from build123d import *

# Parameters (mm, degrees)
SKETCH1_W               = 50
SKETCH1_H               = 6
BOSS_EXTRUDE1_DEPTH     = 8
SKETCH2_W               = 15
SKETCH2_H               = 6
CUT_EXTRUDE1_DEPTH      = 3.1
CUT_EXTRUDE2_DEPTH      = 27.419689627
CUT_EXTRUDE2_DEPTH_BACK = 27.419689627
SKETCH3_R               = 1.6
FILLET1_R               = 2.5


with BuildPart() as part:
    # Sketch1 → Boss-Extrude1 (new, symmetric)
    with BuildSketch(Plane(origin=(0, 0, 0), x_dir=(1, 0, 0), z_dir=(0, 1, 0))):
        Rectangle(SKETCH1_W, SKETCH1_H)
    extrude(amount=BOSS_EXTRUDE1_DEPTH, both=True)

    # Sketch2 → Cut-Extrude1 (cut, symmetric)
    with BuildSketch(Plane(origin=(0, 0, 0), x_dir=(1, 0, 0), z_dir=(0, 1, 0))):
        Polygon((-25, -3), (-10, -3), (-17.736081979, 3), (-25, 3), align=None)
        with Locations((17.5, 0)):
            Rectangle(SKETCH2_W, SKETCH2_H)
        Polygon((5, 3), (-14.736081979, 3), (-7, -3), (5, -3), align=None)
    extrude(amount=CUT_EXTRUDE1_DEPTH, both=True, mode=Mode.SUBTRACT)

    # Sketch3 → Cut-Extrude2 (cut, two sides: drawn at the far end of the back side and taken through both)
    with BuildSketch(Plane(origin=(0, 0, 0), x_dir=(1, 0, 0), z_dir=(0, 1, 0)).offset(-CUT_EXTRUDE2_DEPTH_BACK)):
        with Locations(Location((-22, 0, 0), (0, 0, 270))):
            Circle(SKETCH3_R)
        with Locations(Location((22, 0, 0), (0, 0, 270))):
            Circle(SKETCH3_R)
        with Locations(Location((-2.5, 0, 0), (0, 0, 270))):
            Circle(SKETCH3_R)
    extrude(amount=CUT_EXTRUDE2_DEPTH + CUT_EXTRUDE2_DEPTH_BACK, mode=Mode.SUBTRACT)

    # Fillet1
    fillet1_edges = [part.edges().sort_by_distance(p)[0] for p in [
        (25, -5.55, 3),
        (-25, -5.55, 3),
        (-25, -5.55, -3),
        (25, -5.55, -3),
        (5, 0, -3),
        (5, 0, 3),
        (-14.736081979, 0, -3),
        (10, 0, 3),
        (10, 0, -3),
        (-10, 0, 3),
        (25, 5.55, 3),
        (-25, 5.55, 3),
        (-25, 5.55, -3),
        (25, 5.55, -3),
    ]]
    fillet(fillet1_edges, radius=FILLET1_R - 0.0001)  # a hair under: the kernel refuses the full size


solid = part.part
Work out the finished part from the listing and answer in its coordinate system (mm). A direction names the side the tool comes from. Coordinates: 2 decimals unless noted, no trailing zeros. Write each loop counter-clockwise with the first axis right and the second up, starting at its lowest first coordinate (ties: lowest second). Pieces come first, ordered by that corner, then holes. Notation, with made-up numbers: (2.25, 86.25) - (27.25, 86.25) arc R25 cw to (27.25, 112.25) - close; hole circle Ø8 at (-20, 43). An arc over 180 degrees is marked (long way). One line per question, with ' | ' between items.
1) Consider probe 1 along X at (y, z) = (6.4, 0); probe 2 along Z at (x, y) = (22, 6.4); probe 3 along Y at (x, z) = (-12.5, 2.25). Determine where each line is inside the solid, lowest interval first. Write a range as [from, to].
Checks:
probe 1: [-25, -23.6], [-20.4, -4.1], [-0.9, 20.4], [23.6, 25] | probe 2: [-3, -1.6], [1.6, 3] | probe 3: [-8, -3.1], [3.1, 8]
2) The mould has two halves that part along X. Classify faces 4 (the face through (-10.579, 0.043, 0.224)), 5 (the face through (0, 4, 3)), 6 (the face through (10, 0, 0)): +X half, -X half, draft (parallel to the pull), parting line (faces both ways), or undercut.
Checks:
face 4: undercut | face 5: draft | face 6: +X half
3) Find section B-B, the plane x = 12. Determine the outline of the cut face in (y, z).
Checks:
outline: (-8, -3) - (-3.1, -3) - (-3.1, 3) - (-8, 3) - close; (3.1, -3) - (8, -3) - (8, 3) - (3.1, 3) - close
4) For faces 1 (the face through (-14.79, 0.04, -2.87)), 2 (the face through (-19, 3.1, 1)), 3 (the face through (-4.06, -5.58, -0.35)), determine the directions among +Z, -Z, +X, -X, +Y, -Y from which every point of the face is accessible in a straight line to the end or side of a thin tool.
Checks:
face 1: -Z | face 2: +Z, -X | face 3: +Y, -Y
5) A flat-ended cylindrical pin translates along its axis: P1, Ø0.8, axis at y = -1, z = 0, coming from the -X side. Find the tip coordinate at first contact, or state that the pin passes through.
Checks:
P1: x = -14.38
6) Find section C-C, the plane y = -5.5. Determine the outline of the cut face in (x, z).
Checks:
outline: (-25, -0.5) arc R2.5 ccw to (-22.5, -3) - (22.5, -3) arc R2.5 ccw to (25, -0.5) - (25, 0.5) arc R2.5 ccw to (22.5, 3) - (-22.5, 3) arc R2.5 ccw to (-25, 0.5) - close; hole circle Ø3.2 at (-22, 0); hole circle Ø3.2 at (-2.5, 0); hole circle Ø3.2 at (22, 0)
7) Find section D-D, the plane x = -2.5. Determine the outline of the cut face in (y, z), and give its area (3 significant figures).
Checks:
outline: (-8, -3) - (-3.1, -3) - (-3.1, -1.6) - (-8, -1.6) - close; (-8, 1.6) - (-3.1, 1.6) - (-3.1, 3) - (-8, 3) - close; (3.1, -3) - (8, -3) - (8, -1.6) - (3.1, -1.6) - close; (3.1, 1.6) - (8, 1.6) - (8, 3) - (3.1, 3) - close | area: 27.4 mm2
